Autodesk Inventor part; units mm, degrees
ref_plane "YZ Plane" through (0, 0, 0) normal (1, 0, 0) x (0, 1, 0)
ref_plane "XZ Plane" through (0, 0, 0) normal (0, 1, 0) x (-1, 0, 0)
ref_plane "XY Plane" through (0, 0, 0) normal (0, 0, 1) x (1, 0, 0)
sketch "Sketch1" plane through (0, 0, 0) normal (0, 1, 0) x (-1, 0, 0)
  line L0 (-75.4, 6.25) -> (75.4, 6.25)
  line L1 (78.4, 3.25) -> (78.4, -3.25)
  line L2 (75.4, -6.25) -> (-75.4, -6.25)
  line L3 (-78.4, -3.25) -> (-78.4, 3.25)
  circle A0 centre (-47.65, 0) radius 2.25
  circle A1 centre (47.65, 0) radius 2.25
  circle A2 centre (-47.65, 0) radius 26.75 construction
  circle A3 centre (-10.7, 0) radius 1.7
  circle A4 centre (-10.7, 0) radius 11.2 construction
  line L4 (-21.9, 0) -> (-21.9, 5.3604)
  line L5 (-20.9, 0) -> (-20.9, 5.3604)
  circle A5 centre (10.7, 0) radius 2.25
  circle A6 centre (10.7, 0) radius 11.2 construction
  line L6 (-0.5, 0) -> (-0.5, 4.194)
  line L7 (0.5, 0) -> (0.5, 4.194)
  circle A7 centre (47.65, 0) radius 26.75 construction
  line L8 (20.9, 0) -> (20.9, 4.3426)
  line L9 (21.9, 0) -> (21.9, 4.3426)
  arc A8 (-75.4, 6.25) -> (-78.4, 3.25) centre (-75.4, 3.25) ccw
  arc A9 (-78.4, -3.25) -> (-75.4, -6.25) centre (-75.4, -3.25) ccw
  arc A10 (78.4, 3.25) -> (75.4, 6.25) centre (75.4, 3.25) ccw
  arc A11 (75.4, -6.25) -> (78.4, -3.25) centre (75.4, -3.25) ccw
  line L10 (-81.9483, 0) -> (78.4, 0) construction
  circle A12 centre (-10.7, 0) radius 13.2
  circle A13 centre (-10.7, 0) radius 17.7
  line L11 (74.4, 0) -> (74.4, 11.2)
  line L12 (-74.4, 0) -> (-74.4, 10)
  line L13 (-75.4, 20) -> (-74.4, 20)
  line L14 (-71.4, 17) -> (-71.4, -17)
  line L15 (-74.4, -20) -> (-75.4, -20)
  line L16 (-78.4, -17) -> (-78.4, 17)
  line L17 (75.4, 20) -> (74.4, 20)
  line L18 (71.4, 17) -> (71.4, -17)
  line L19 (74.4, -20) -> (75.4, -20)
  line L20 (78.4, -17) -> (78.4, 17)
  arc A14 (74.4, 20) -> (71.4, 17) centre (74.4, 17) ccw
  arc A15 (78.4, 17) -> (75.4, 20) centre (75.4, 17) ccw
  arc A16 (75.4, -20) -> (78.4, -17) centre (75.4, -17) ccw
  arc A17 (71.4, -17) -> (74.4, -20) centre (74.4, -17) ccw
  arc A18 (-75.4, 20) -> (-78.4, 17) centre (-75.4, 17) ccw
  arc A19 (-71.4, 17) -> (-74.4, 20) centre (-74.4, 17) ccw
  arc A20 (-74.4, -20) -> (-71.4, -17) centre (-74.4, -17) ccw
  arc A21 (-78.4, -17) -> (-75.4, -20) centre (-75.4, -17) ccw
  line L21 (-19.3726, 23.4692) -> (-1.7741, 23.4692)
  line L22 (-1.7741, 23.4692) -> (-1.7741, 7.4894)
  line L23 (-1.7741, 7.4894) -> (-19.3726, 7.4894)
  line L24 (-19.3726, 7.4894) -> (-19.3726, 23.4692)
  point P0 (0, 0)
  point P1 (-78.4, 6.25)
  point P2 (-78.4, -6.25)
  point P3 (0, 6.25)
  point P4 (-78.4, 20)
  point P5 (-71.4, 20)
  point P6 (-78.4, -20)
  point P7 (-78.4, 0)
  point P8 (-78.4, 0)
  point P9 (78.4, 20)
  point P10 (71.4, 20)
  point P11 (78.4, -20)
  point P12 (78.4, 0)
  dimension "d0" = 12.5
  dimension "d1" = 4.5
  dimension "d3" = 4.5
  dimension "d5" = 53.5
  dimension "d6" = 3.4
  dimension "d7" = 22.4
  dimension "d8" = 1
  dimension "d9" = 4.5
  dimension "d10" = 22.4
  dimension "d11" = 1
  dimension "d12" = 53.5
  dimension "d13" = 1
  dimension "d14" = 3
  dimension "d23" = 4.5
  dimension "d26" = 4
  dimension "d27" = 4
  dimension "d28" = 7
  dimension "d29" = 40
  dimension "d30" = 7
  dimension "d31" = 40
  dimension "d32" = 3
  dimension "d33" = 3
  dimension "d39" = 2
extrude "Extrusion1" add sketch "Sketch1" along normal blind 3 contours A8 L16 A18 L13 A19 L14 L0 | L0 L14 L2 A9 L3 A8 | L0 A13 L2 L14 | A9 L2 L14 A20 L15 A21 L16 | A13 L24 A12 L0 | L0 A12 L2 A13 | A13 L22 A12 L24 | L2 A12 A13 | A12 L22 A13 L0 | L0 A13 L2 A12 | A13 L0 L18 L2 | L18 L0 A10 L1 A11 L2 | L2 A11 L20 A16 L19 A17 L18 | L18 A14 L17 A15 L20 A10 L0
extrude "Extrusion2" cut sketch "Sketch1" along normal blind 10 contours A12 L24 L23 L22 L0 | L0 A12 L2 | A12 L22 L23 L24 | L2 A12
sketch "Sketch2" plane through (0, 3, 0) normal (0, 1, 0) x (1, 0, 0)
  circle A0 centre (47.65, 0) radius 2.25
  circle A1 centre (-10.7, 0) radius 2.25
  circle A2 centre (-47.65, 0) radius 2.25
  circle A3 centre (-47.65, 0) radius 12.25
  circle A4 centre (-10.7, 0) radius 12.25
  circle A5 centre (47.65, 0) radius 12.25
  point P0 (0, 0)
  dimension "d34" = 10
  dimension "d35" = 10
  dimension "d36" = 10
extrude "Extrusion3" add sketch "Sketch2" along normal blind 3
extrude "Extrusion4" cut sketch "Sketch1" along normal blind 3 contours L24 L21 L22 A13 | A13 L22 A12 L24 | A12 L22 L23 L24
extrude "Extrusion5" add sketch "Sketch2" against normal blind 3
extrude "Extrusion6" cut sketch "Sketch1" along normal mid plane 20 contours A12 L24 L23 L22 L0 | L0 A12 L2 | A12 L22 L23 L24 | L2 A12
equation "\"sp\" = 0.4"
properties part number "OuterBar"
Here's how the part is built. I have some questions about the finished solid (model axes, mm). A direction names the side the tool comes from. Coordinates: 2 decimals unless noted, no trailing zeros. Order: outer loops, then holes, each group sorted by start corner. A loop starts at its lowest first (then second) coordinate and runs counter-clockwise, first axis right, second up. Notation, with made-up numbers: (55.5, 46) - (100.5, 46) arc R14 ccw to (100.5, 72) - close; hole circle Ø2 at (41.25, 58). An arc over 180 degrees is marked (long way). One line per question, with ' | ' between items. Start each with the question number.
1. If we section it at A-A (y = 2): Give the number of separate pieces and of enclosed holes in the cut face, and give its area (3 significant figures).
2. Please list where these lines run through material, in increasing order: line 1 along X through (y, z) = (2.2, 0); line 2 along Z through (x, y) = (47.65, 2.65); line 3 along X through (y, z) = (3.8, -6). Write a range as [from, to].
3. I'm going to push flat-ended pins straight in: pin 1 Ø10 at (x, z) = (17, 13) entering from +Y; pin 2 Ø2.5 at (x, y) = (64, 1.5) entering from +Z; pin 3 Ø0.9 at (x, y) = (63.5, 1) entering from -Z; pin 4 Ø4 at (x, z) = (-47.65, 0) entering from -Y. Where does each tip first touch, or does it pass through?
4. If we mould it in two halves opening along Z, with no side actions, what happens to faces 5 (the cylindrical face through (47.798, 3.625, 2.245)), 6 (the flat face through (71, 3, 0)), 7 (the cylindrical face through (-77.54, 1.48, -19.1))? For each: released by +Z, released by -Z, zero draft, split by the parting line, or undercut.
5. If we section it at B-B (x = 10.7): Write out the boundary of the cut face in (y, z), and give its area (3 significant figures).
6. Which directions (+Z, -Z, +X, -X, +Y, -Y) give clear straight access to the entire face, cutting with the end or side of a thin tool? Please do faces 1 (the cylindrical face through (72.3, 1.48, 19.14)), 2 (the flat face through (0, 3, 11)), 3 (the cylindrical face through (-59.89, 3.62, 0.54)), 4 (the flat face through (32, 1, -6.25)).
Model answer:
1) separate pieces: 1 | enclosed holes: 3 | area: 2,710 mm²
2) line 1: x = [-78.4, -49.9], [-45.4, -12.95], [-8.45, -2.5], [23.9, 45.4], [49.9, 78.4] | line 2: z = [-12.25, -2.25], [2.25, 12.25] | line 3: x = [-58.33, -36.97], [-21.38, -1.06], [36.97, 58.33]
3) pin 1: stops at y = 3 | pin 2: stops at z = 6.25 | pin 3: stops at z = -6.25 | pin 4: passes through
4) face 5: undercut | face 6: zero draft | face 7: released by -Z
5) outline: (0, -17.7) - (3, -17.7) - (3, -13.2) - (0, -13.2) - close | area: 13.5 mm²
6) face 1: +Z, +Y, -Y | face 2: +Z, +Y | face 3: +Y | face 4: -Z, +Y, -Y
